Could you check a few things on this model? Use its own coordinates, in mm. A direction names the side the tool comes from. Round coordinates to 2 decimals unless told otherwise and drop trailing zeros. Write each loop counter-clockwise with the first axis right and the second up, starting at its lowest first coordinate (ties: lowest second). Pieces come first, ordered by that corner, then holes. Notation, with made-up numbers: (66, -17) - (72, -17) arc R20 cw to (72, -7) - close; hole circle Ø1 at (31, 74). An arc over 180 degrees is marked (long way). Put each result on its own line as item: value.
from build123d import *

# Parameters (mm, degrees)
F0_W     = 2438.4
F0_H     = 101.6
F1_DEPTH = 38.1
F3_DEPTH = 3.175


with BuildPart() as f1:
    # F0 (on Front) → F1 (new body)
    with BuildSketch(Plane.XZ):
        with Locations((0, 63.5)):
            Rectangle(F0_W, F0_H)
    extrude(amount=F1_DEPTH)



with BuildPart() as f1b:
    # F0 (on Front) → F1, piece 2 (new body)
    with BuildSketch(Plane.XZ):
        with Locations((0, -50.8)):
            Rectangle(F0_W, F0_H)
    extrude(amount=F1_DEPTH)


with BuildPart() as f1c:
    # F0 (on Front) → F1, piece 3 (new body)
    with BuildSketch(Plane.XZ):
        with Locations((0, -165.1)):
            Rectangle(F0_W, F0_H)
    extrude(amount=F1_DEPTH)


with BuildPart() as f1_1:
    add(f1.part)

    add(f1b.part)  # F3 merges F1b

    add(f1c.part)  # F3 merges F1c
    # F2 (on face) → F3 (join)
    with BuildSketch(Plane.XZ.offset(38.1)):
        with BuildLine():
            Line((-1212.85, 41.9409019501), (-1212.85, -152.4))
            ThreePointArc((-1212.85, -152.4), (-1162.05, -203.2), (-1111.25, -152.4))
            Line((-1111.25, -152.4), (-1111.25, 41.9409019501))
            ThreePointArc((-1111.25, 41.9409019501), (-1162.05, 92.7409019501), (-1212.85, 41.9409019501))
        make_face()
        with BuildLine():
            Line((1111.25, 41.9409019501), (1111.25, -152.4))
            ThreePointArc((1111.25, -152.4), (1162.05, -203.2), (1212.85, -152.4))
            Line((1212.85, -152.4), (1212.85, 41.9409019501))
            ThreePointArc((1212.85, 41.9409019501), (1162.05, 92.7409019501), (1111.25, 41.9409019501))
        make_face()
    extrude(amount=F3_DEPTH)


solid = f1_1.part
(1) Imagine slicing it at A-A, the plane x = 1040. List the corners of the cut face in (y, z) for me, then the cut area to 3 significant figures.
Values found:
outline: (-38.1, -215.9) - (0, -215.9) - (0, -114.3) - (-38.1, -114.3) - close; (-38.1, -101.6) - (0, -101.6) - (0, 0) - (-38.1, 0) - close; (-38.1, 12.7) - (0, 12.7) - (0, 114.3) - (-38.1, 114.3) - close
area: 11,600 mm^2
(2) Please list where these lines run through material, in increasing order: probe 1 along Z at (x, y) = (-251, -30.5); probe 2 along Y at (x, z) = (982.5, 17.5); probe 3 along X at (y, z) = (-38.5, 70.5). Write a range as from..to.
Values found:
probe 1: z = -215.9..-114.3, -101.6..0, 12.7..114.3
probe 2: y = -38.1..0
probe 3: x = -1204.06..-1120.04, 1120.04..1204.06
(3) I'm going to push flat-ended pins straight in: pin 1 (10 mm diameter, centred on x = 1150.5, z = 6.5, fed in from +Y); pin 2 (1 mm diameter, centred on y = -40.5, z = -90, fed in from +X); pin 3 (1.9 mm diameter, centred on x = -1217, z = -68.5, fed in from -Y). Where does each tip first touch, or does it pass through?
Values found:
pin 1: stops at y = -38.1
pin 2: stops at x = 1212.85
pin 3: stops at y = -38.1
(4) For faces 1 (the face through (1160.933, -39.665, -203.188)), 2 (the face through (1163.17, -39.67, 92.73)), 3 (the face through (-1219.2, -19, -52)), which set-ups out of +Z, -Z, +X, -X, +Y, -Y let a thin tool reach every point of the face, with its end or its side?
Values found:
face 1: -Z, -Y
face 2: +Z, -Y
face 3: +Z, -Z, -X, +Y, -Y
(5) Imagine slicing it at B-B, the plane y = -22. List the corners of the cut face in (x, z) for me, then the cut area to 3 significant figures.
Values found:
outline: (-1219.2, -215.9) - (1219.2, -215.9) - (1219.2, -114.3) - (-1219.2, -114.3) - close; (-1219.2, -101.6) - (1219.2, -101.6) - (1219.2, 0) - (-1219.2, 0) - close; (-1219.2, 12.7) - (1219.2, 12.7) - (1219.2, 114.3) - (-1219.2, 114.3) - close
area: 743,000 mm^2
(6) Imagine slicing it at C-C, the plane z = -26. List the corners of the cut face in (x, y) for me (3 decimals), then the cut area to 3 significant figures.
Values found:
outline: (-1219.2, -38.1) - (-1212.85, -38.1) - (-1212.85, -41.275) - (-1111.25, -41.275) - (-1111.25, -38.1) - (1111.25, -38.1) - (1111.25, -41.275) - (1212.85, -41.275) - (1212.85, -38.1) - (1219.2, -38.1) - (1219.2, 0) - (-1219.2, 0) - close
area: 93,500 mm^2
